Can you work these out from the model? Positions are in its coordinate system, mm. Face numbers are marked on the shaded views. A direction names the side the tool comes from. Round coordinates to 2 decimals unless told otherwise and drop trailing zeros. Loops run counter-clockwise (first coordinate to the right, second up) from the corner with the lowest first, then second, coordinate; pieces in that order, holes last.
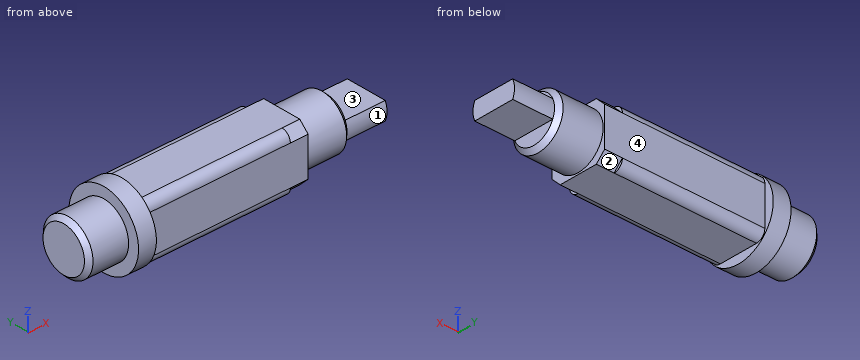
from build123d import *

# Parameters (mm, degrees)
EXTRUDE_1_DEPTH = 16
EXTRUDE_2_DEPTH = 2
EXTRUDE_3_DEPTH = 5


with BuildPart() as part:
    # 草图1 → 旋转1 (revolve)
    with BuildSketch(Plane.XY):
        Polygon((0, 3), (4, 3), (4, 4.2), (6, 4.2), (6, 0), (0, 0), (-0.5, 0), (-0.5, 2.5), align=None)
    revolve(axis=Axis((6, 0, 0), (-1, 0, 0)))

    # 草图2 → 凸台-拉伸1 (add)
    with BuildSketch(Plane(origin=(6, 0, 0), x_dir=(0, 0, -1), z_dir=(1, 0, 0))):
        with BuildLine():
            Line((-2.181980515, 3.181980515), (2.181980515, 3.181980515))
            ThreePointArc((2.181980515, 3.181980515), (2.889087297, 2.889087297), (3.181980515, 2.181980515))
            Line((3.181980515, 2.181980515), (3.181980515, -2.181980515))
            ThreePointArc((3.181980515, -2.181980515), (2.889087297, -2.889087297), (2.181980515, -3.181980515))
            Line((2.181980515, -3.181980515), (-2.181980515, -3.181980515))
            ThreePointArc((-2.181980515, -3.181980515), (-2.889087297, -2.889087297), (-3.181980515, -2.181980515))
            Line((-3.181980515, -2.181980515), (-3.181980515, 2.181980515))
            ThreePointArc((-3.181980515, 2.181980515), (-2.889087297, 2.889087297), (-2.181980515, 3.181980515))
        make_face()
    extrude(amount=EXTRUDE_1_DEPTH)

    # 草图3 → 凸台-拉伸2 (add)
    with BuildSketch(Plane(origin=(22, 0, 0), x_dir=(0, 0, -1), z_dir=(1, 0, 0))):
        Polygon((3.181980515, 2.181980515), (2.181980515, 3.181980515), (-2.181980515, 3.181980515), (-3.181980515, 2.181980515), (-3.181980515, -2.181980515), (-2.181980515, -3.181980515), (2.181980515, -3.181980515), (3.181980515, -2.181980515), align=None)
    extrude(amount=EXTRUDE_2_DEPTH)

    # 草图4 → 旋转2 (revolve)
    with BuildSketch(Plane.XY):
        Polygon((28.5, 3), (29, 2.5), (29, 0), (24, 0), (24, 3), align=None)
    revolve(axis=Axis((29, 0, 0), (-1, 0, 0)))

    # 草图5 → 凸台-拉伸3 (add)
    with BuildSketch(Plane(origin=(28.5, 0, 0), x_dir=(0, 0, -1), z_dir=(1, 0, 0))):
        with BuildLine():
            Line((-1, -1.791287847), (-1, -2.291287847))
            ThreePointArc((-1, -2.291287847), (0, -2.5), (1, -2.291287847))
            Line((1, -2.291287847), (1, -1.791287847))
            Line((1, -1.791287847), (1, 1.791287847))
            Line((1, 1.791287847), (1, 2.291287847))
            ThreePointArc((1, 2.291287847), (0, 2.5), (-1, 2.291287847))
            Line((-1, 2.291287847), (-1, 1.791287847))
            Line((-1, 1.791287847), (-1, -1.791287847))
        make_face()
    extrude(amount=EXTRUDE_3_DEPTH)


solid = part.part
(1) For the marked faces 1, 2, 3 and 4, which set-ups out of +Z, -Z, +X, -X, +Y, -Y let a thin tool reach every point of the face, with its end or its side?
Worked answers:
face 1: +X, -Y
face 2: -Z, +X, +Y
face 3: +Z, +X, +Y, -Y
face 4: +Z, -Z, +X, +Y
(2) If we section it at D-D, the plane x = 23: List the corners of the cut face in (y, z) for me.
Worked answers:
outline: (-3.18, -2.18) - (-2.18, -3.18) - (2.18, -3.18) - (3.18, -2.18) - (3.18, 2.18) - (2.18, 3.18) - (-2.18, 3.18) - (-3.18, 2.18) - close
(3) If I drill on line 1 (Y direction, x = 12, z = 1.5); line 2 (X direction, y = 1.75, z = -3), over which ranges is the centre line in solid material (lowest first)?
Worked answers:
line 1: y = -3.18 to 3.18
line 2: x = 4 to 24
(4) If we section it at C-C, the plane y = 0: List the corners of the cut face in (x, z) for me, then the cut area to 3 significant figures.
Worked answers:
outline: (-0.5, -2.5) - (0, -3) - (4, -3) - (4, -4.2) - (6, -4.2) - (6, -3.18) - (24, -3.18) - (24, -3) - (28.5, -3) - (29, -2.5) - (29, -1) - (33.5, -1) - (33.5, 1) - (29, 1) - (29, 2.5) - (28.5, 3) - (24, 3) - (24, 3.18) - (6, 3.18) - (6, 4.2) - (4, 4.2) - (4, 3) - (0, 3) - (-0.5, 2.5) - close
area: 197 mm2
(5) Will these pins go through, and if not, where does the flat tip stop? P1, Ø5, axis at x = 13, z = 1, coming from the -Y side; P2, Ø1.3, axis at x = 13.5, y = 0, coming from the +Z side; P3, Ø5, axis at x = 32, y = -0.5, coming from the -Z side; P4, Ø1.2, axis at y = 0, z = -1.5, coming from the +X side.
Worked answers:
P1: stops at y = -3.18
P2: stops at z = 3.18
P3: stops at z = -1
P4: stops at x = 33.5
(6) If we section it at B-B, the plane z = 0: List the corners of the cut face in (x, y) for me.
Worked answers:
outline: (-0.5, -2.5) - (0, -3) - (4, -3) - (4, -4.2) - (6, -4.2) - (6, -3.18) - (24, -3.18) - (24, -3) - (28.5, -3) - (29, -2.5) - (33.5, -2.5) - (33.5, 2.5) - (29, 2.5) - (28.5, 3) - (24, 3) - (24, 3.18) - (6, 3.18) - (6, 4.2) - (4, 4.2) - (4, 3) - (0, 3) - (-0.5, 2.5) - close
(7) If we section it at A-A, the plane x = 7.5: List the corners of the cut face in (y, z) for me.
Worked answers:
outline: (-3.18, -2.18) arc R1 ccw to (-2.18, -3.18) - (2.18, -3.18) arc R1 ccw to (3.18, -2.18) - (3.18, 2.18) arc R1 ccw to (2.18, 3.18) - (-2.18, 3.18) arc R1 ccw to (-3.18, 2.18) - close
